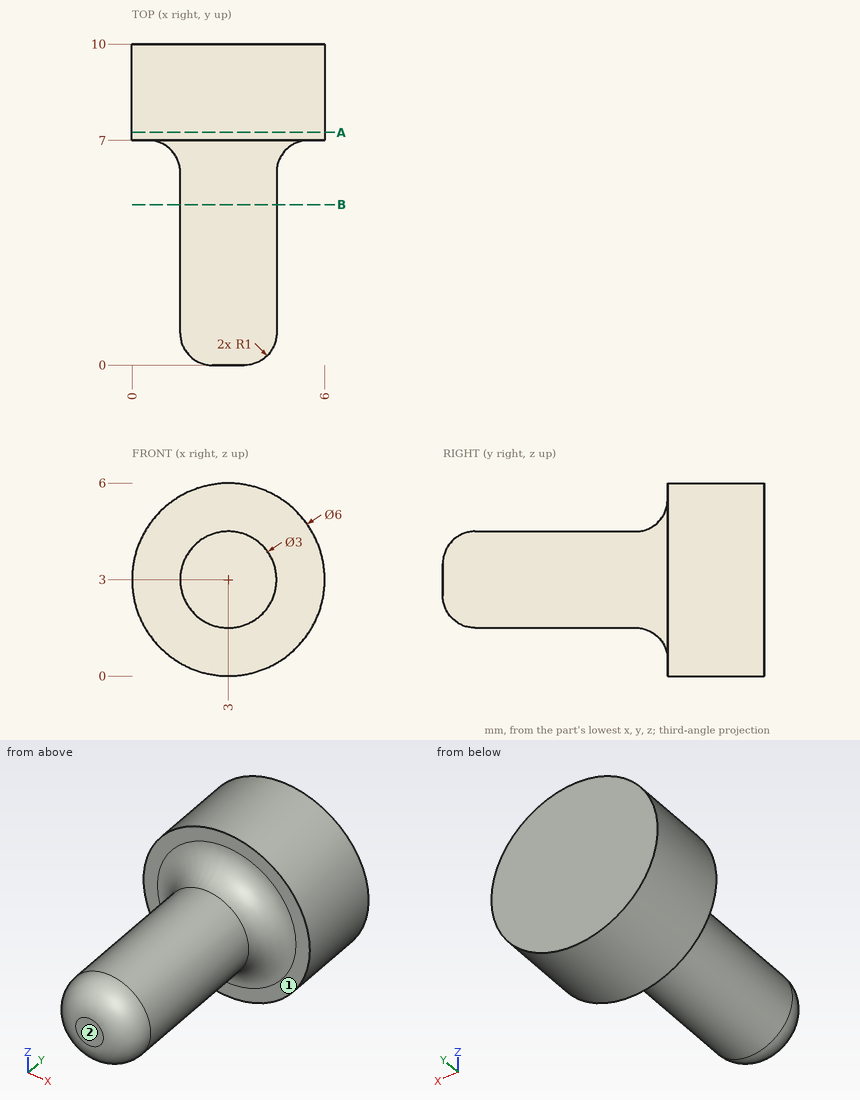
Verification items for this drawing (mm, ordinates from the low corner). A direction names the side the tool comes from. Give positions to 0.01 mm unless a question says otherwise; leave off trailing zeros. Write each loop counter-clockwise with the first axis right and the second up, starting at its lowest first coordinate (ties: lowest second). Pieces come first, ordered by that corner, then holes. Notation, with made-up numbers: (75.25, -31) - (100.25, -31) arc R19 ccw to (100.25, 4) - close; hole circle Ø2 at (57.25, -20). An arc over 180 degrees is marked (long way). Answer as a JSON object with one key per item and string values. Group by question number.
1) Access from +Z, -Z, +X, -X, +Y, -Y to the whole of each face (thin tool, end or side, straight path). Record for the marked faces 1 and 2.
2) Depth check by flat-ended pin: P1, Ø3, axis at x = 1, y = 3.5, coming from the -Z side; P2, Ø1, axis at y = 8, z = 3.5, coming from the -X side; P3, Ø2, axis at x = 4.5, y = 6.5, coming from the +Z side; P4, Ø1, axis at x = 4.5, y = 8, coming from the -Z side. Enter the tip coordinate at first touch or a pass-through.
3) Sectioned sample at A-A (y = 7.25). Record the cut outline in (x, z), then the cut area to 3 significant figures.
4) Sectioned sample at B-B (y = 5). Record the cut outline in (x, z).
5) Thickness scan on probe 1 along Y at (x, z) = (5.05, 4.4); probe 2 along Z at (x, y) = (3.7, 5); probe 3 along Y at (x, z) = (4.1, 4.35). Record the ranges inside material, lowest first. Write a range as from..to.
Geometry results:
{
 "1": {"face 1": "-Y", "face 2": "+Z, -Z, +X, -X, -Y"},
 "2": {"P1": "stops at z = 1.59", "P2": "stops at x = 0", "P3": "stops at z = 5.93", "P4": "stops at z = 0.17"},
 "3": {"outline": "circle Ø6 at (3, 3)", "area": "28.3 mm^2"},
 "4": {"outline": "circle Ø3 at (3, 3)"},
 "5": {"probe 1": "y = 7..10", "probe 2": "z = 1.67..4.33", "probe 3": "y = 6.65..10"}
}
